Could you check a few things on this drawing? It's one solid part, dimensions in mm from its lowest x, y, z. Coordinates: 2 decimals unless noted, no trailing zeros. Order: outer loops, then holes, each group sorted by start corner. A loop starts at its lowest first (then second) coordinate and runs counter-clockwise, first axis right, second up.
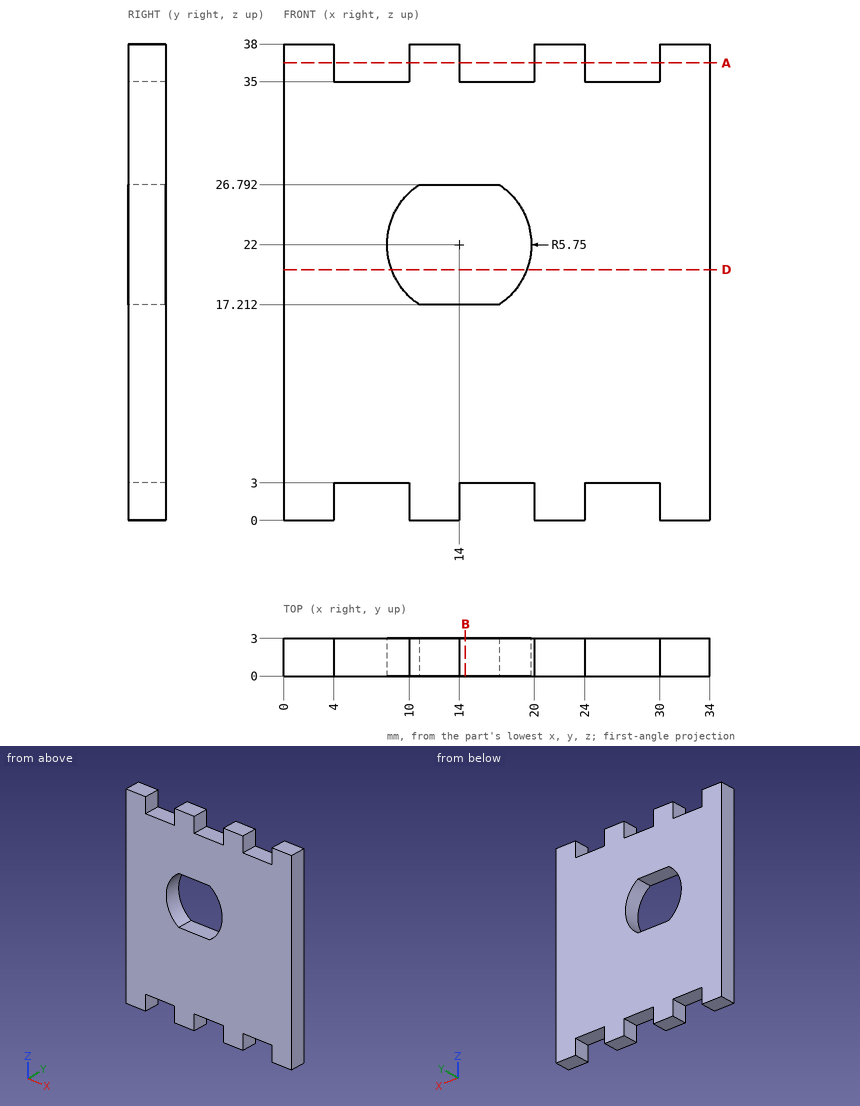
Q1. If we section it at D-D on z = 20: Write out the boundary of the cut face in (x, y).
Q2. If we section it at B-B on x = 14.5: Write out the boundary of the cut face in (y, z).
Q3. If we section it at A-A on z = 36.5: Write out the boundary of the cut face in (x, y), then the cut area to 3 significant figures.
Q4. I need wall thicknesses on L1, parallel to Z at x = 13, y = 2.05; L2, parallel to Z at x = 6.5, y = 1.2; L3, parallel to X at y = 2.75, z = 18.5. Which ranges of each line are inside material? Lowest first, please.
Q5. Will these pins go through, and if not, where does the flat tip stop? pin 1 (1.5 mm diameter, centred on y = 2, z = 36, fed in from -X); pin 2 (0.9 mm diameter, centred on x = 18.5, y = 1.5, fed in from +Z); pin 3 (1.5 mm diameter, centred on x = 15.5, y = 1, fed in from -Z).
Reply:
1. outline: (0, 0) - (8.61, 0) - (8.61, 3) - (0, 3) - close; (19.39, 0) - (34, 0) - (34, 3) - (19.39, 3) - close
2. outline: (0, 3) - (3, 3) - (3, 17.21) - (0, 17.21) - close; (0, 26.79) - (3, 26.79) - (3, 35) - (0, 35) - close
3. outline: (0, 0) - (4, 0) - (4, 3) - (0, 3) - close; (10, 0) - (14, 0) - (14, 3) - (10, 3) - close; (20, 0) - (24, 0) - (24, 3) - (20, 3) - close; (30, 0) - (34, 0) - (34, 3) - (30, 3) - close
3. area: 48.0 mm2
4. L1: z = 0 to 17.21, 26.79 to 38
4. L2: z = 3 to 35
4. L3: x = 0 to 9.44, 18.56 to 34
5. pin 1: stops at x = 0
5. pin 2: stops at z = 35
5. pin 3: stops at z = 3
